Autodesk Fusion 360 part; units mm, degrees
sketch "Sketch1" plane through (0, 0, 0) normal (0, 1, 0) x (1, 0, 0)
  line L0 (0, 0) -> (0, -88)
  line L1 (0, -88) -> (47, -88)
  line L2 (47, -88) -> (47, -80)
  line L3 (47, -80) -> (43, -80)
  line L4 (43, -80) -> (43, -76)
  line L5 (43, -76) -> (47, -76)
  line L6 (47, -76) -> (47, -72)
  line L7 (47, -72) -> (43, -72)
  line L8 (43, -72) -> (43, -68)
  line L9 (43, -68) -> (47, -68)
  line L10 (47, -68) -> (47, -64)
  line L11 (47, -64) -> (43, -64)
  line L12 (43, -64) -> (43, -60)
  line L13 (43, -60) -> (47, -60)
  line L14 (47, -60) -> (47, -0.077)
  line L15 (47, -0.077) -> (41, -0.077)
  line L16 (41, -0.077) -> (41, -80)
  line L17 (41, -80) -> (0, -80)
  dimension "d1" = 88
  dimension "d2" = 47
  dimension "d3" = 8
  dimension "d4" = 4
  dimension "d5" = 4
  dimension "d6" = 4
  dimension "d7" = 4
  dimension "d8" = 4
  dimension "d9" = 4
  dimension "d10" = 4
  dimension "d11" = 4
  dimension "d12" = 4
  dimension "d13" = 4
  dimension "d14" = 4
  dimension "d16" = 6
revolve "Revolve1" add sketch "Sketch1" angle 360 about axis through (0, 0, 0) along (0, 0, 1)
sketch "Sketch2" plane through (0, 0, 0) normal (0, 1, 0) x (1, 0, 0)
  line L0 (-46.9446, 0) -> (-39.667, 0)
  line L1 (-21.667, -18) -> (0, -18)
  line L2 (0, 0) -> (0, -37.5033) construction
  arc A0 (-39.667, 0) -> (-21.667, -18) centre (-21.667, 0) ccw
  line L3 (21.667, -18) -> (0, -18)
  arc A1 (21.667, -18) -> (39.667, 0) centre (21.667, 0) ccw
  circle A2 centre (0, -44) radius 10
  line L4 (-39.667, 0) -> (39.667, 0)
  point P0 (-39.667, -18)
  dimension "d17" = 18
  dimension "d18" = 18
  dimension "d19" = 20
  dimension "d20" = 44
extrude "Extrude1" cut sketch "Sketch2" along normal mid plane 180
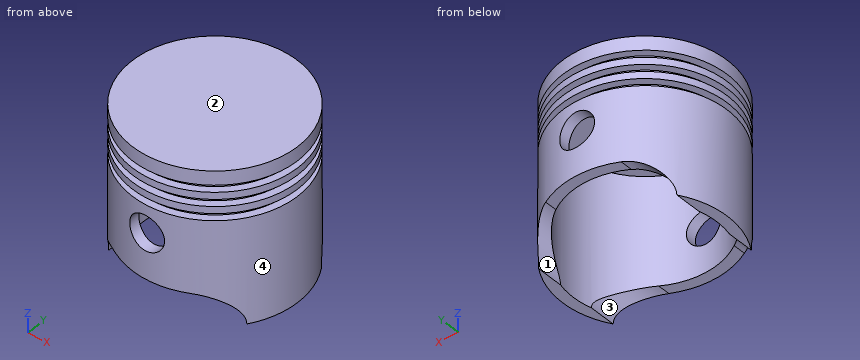
Can you work these out from the model? Positions are in its coordinate system, mm. Face numbers are marked on the shaded views. Round coordinates to 2 decimals unless told otherwise and drop trailing zeros. Order: outer loops, then holes, each group sorted by start corner. A loop starts at its lowest first (then second) coordinate and runs counter-clockwise, first axis right, second up. Notation, with made-up numbers: (-12, -23.75) -> (46, -23.75) arc R10 ccw to (46, -8.75) -> close; hole circle Ø10 at (-8, 58.25). An arc over 180 degrees is marked (long way). Write each question's results on one line, items separated by ' | '. Start each with the question number.
Item 1: If we section it at A-A, the plane z = 44: Write out the boundary of the cut face in (x, y), then the cut area to 3 significant figures.
Item 2: If we section it at C-C, the plane z = 32: Write out the boundary of the cut face in (x, y), then the cut area to 3 significant figures.
Item 3: Please list where these lines run through material, in increasing order: L1, parallel to Z at x = 0, y = -45; L2, parallel to Z at x = 0, y = 42.5; L3, parallel to Z at x = 27, y = 25.5.
Item 4: If we section it at B-B, the plane x = 0: State how many separate pieces and enclosed holes the cut face has, then the cut area to 3 significant figures.
Item 5: Will these pins go through, and if not, where does the flat tip stop? pin 1 (2 mm diameter, centred on x = -1, y = 23.5, fed in from -Z); pin 2 (1.5 mm diameter, centred on y = 3, z = 59, fed in from +X); pin 3 (4 mm diameter, centred on x = -10.5, z = 60.5, fed in from -Y); pin 4 (23 mm diameter, centred on x = 0, z = 44, fed in from -Y).
Item 6: Thinking about a two-plate mould opening in X: for the marked faces 1, 2, 3 and 4, which applies, +X half, -X half, draft (parallel to the pull), parting line (faces both ways), or undercut?
Results:
1) outline: (-10, -45.92) -> (-10, -39.76) arc R41 cw to (-10, 39.76) -> (-10, 45.92) arc R47 ccw to start; (10, -45.92) arc R47 ccw to (10, 45.92) -> (10, 39.76) arc R41 cw to (10, -39.76) -> close | area: 1,420 mm2
2) outline: circle Ø94 at (0, 0); hole circle Ø82 at (0, 0) | area: 1,660 mm2
3) L1: z = 18 to 34, 54 to 60, 64 to 68, 72 to 76, 80 to 88 | L2: z = 18 to 34, 54 to 88 | L3: z = 80 to 88
4) separate pieces: 3 | enclosed holes: 0 | area: 1,160 mm2
5) pin 1: stops at z = 80 | pin 2: stops at x = 46.95 | pin 3: stops at y = -46.21 | pin 4: stops at y = -47
6) face 1: undercut | face 2: draft | face 3: undercut | face 4: parting line
